Geometry check sheet. Reference: the model listing, model coordinates, mm. Face numbers are marked on the shaded views. A direction names the side the tool comes from. Give positions to 0.01 mm unless a question says otherwise; leave off trailing zeros. Loops run counter-clockwise (first coordinate to the right, second up) from the corner with the lowest first, then second, coordinate; pieces in that order, holes last. Notation, with made-up numbers: (52.5, 56.25) -> (82.5, 56.25) arc R32 ccw to (82.5, 82.25) -> close; hole circle Ø8 at (31.25, 70.5). An arc over 180 degrees is marked (long way). One line per question, with ' | ' between items.
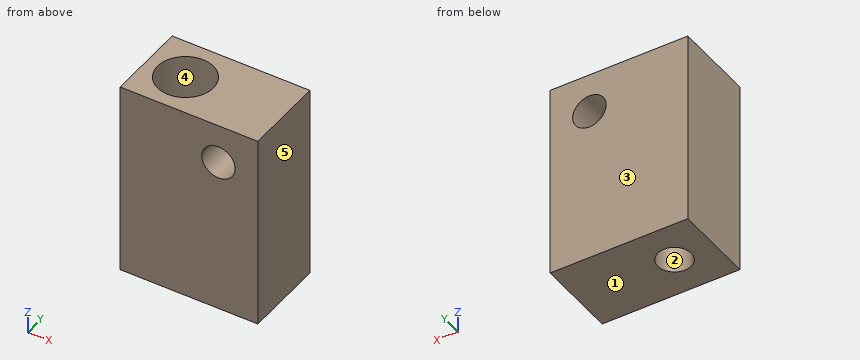
from build123d import *

# Parameters (mm, degrees)
F0_W     = 42
F0_H     = 60
F1_DEPTH = 25
F4_D     = 10.2
F4_DEPTH = 100
F4_TIP   = 3.064389157
F5_D     = 10.2
F5_DEPTH = 100
F5_TIP   = 3.064389157
F6_D     = 17
F6_DEPTH = 35
F6_TIP   = 5.1073152617


with BuildPart() as f1:
    # F0 (on Front) → F1 (new body)
    with BuildSketch(Plane.XZ):
        with Locations((-52.5741710365, 48.0550478399)):
            Rectangle(F0_W, F0_H)
    extrude(amount=F1_DEPTH)

    # F4
    with Locations(Plane.XZ.offset(25)):
        with Locations((-43.5741710365, 66.0550478399)):
            Hole(F4_D / 2, depth=F4_DEPTH)
            with Locations((0, 0, -(F4_DEPTH + F4_TIP / 2))):  # 118° drill point
                Cone(0, F4_D / 2, F4_TIP, mode=Mode.SUBTRACT)

    # F5
    with Locations(Plane.XY.offset(78.0550478399)):
        with Locations((-61.5741710365, -12.5)):
            Hole(F5_D / 2, depth=F5_DEPTH)
            with Locations((0, 0, -(F5_DEPTH + F5_TIP / 2))):  # 118° drill point
                Cone(0, F5_D / 2, F5_TIP, mode=Mode.SUBTRACT)

    # F6
    with Locations(Plane.XY.offset(78.0550478399)):
        with Locations((-61.5741710365, -12.5)):
            Hole(F6_D / 2, depth=F6_DEPTH)
            with Locations((0, 0, -(F6_DEPTH + F6_TIP / 2))):  # 118° drill point
                Cone(0, F6_D / 2, F6_TIP, mode=Mode.SUBTRACT)


solid = f1.part
Item 1: Scan lines: probe 1 along X at (y, z) = (-12.5, 34.25); probe 2 along X at (y, z) = (-12.5, 53.5); probe 3 along X at (y, z) = (-8.25, 69). Record each from-to range of solid material in increasing order.
Result:
probe 1: -73.57 to -66.67, -56.47 to -31.57 | probe 2: -73.57 to -70.07, -53.07 to -31.57 | probe 3: -73.57 to -68.94, -54.21 to -47.74, -39.41 to -31.57
Item 2: Sectioned sample at A-A (y = -12.5). Record the cut outline in (x, z), plus the area to 3 significant figures.
Result:
outline: (-73.57, 18.06) -> (-66.67, 18.06) -> (-66.67, 41.01) -> (-70.07, 43.06) -> (-70.07, 78.06) -> (-73.57, 78.06) -> close; (-56.47, 18.06) -> (-31.57, 18.06) -> (-31.57, 78.06) -> (-53.07, 78.06) -> (-53.07, 43.06) -> (-56.47, 41.01) -> close; hole circle Ø10.2 at (-43.57, 66.06) | area: 1,580 mm2
Item 3: Sectioned sample at C-C (x = -43). Record the cut outline in (y, z), plus the area to 3 significant figures.
Result:
outline: (-25, 18.06) -> (0, 18.06) -> (0, 60.99) -> (-25, 60.99) -> close; (-25, 71.12) -> (0, 71.12) -> (0, 78.06) -> (-25, 78.06) -> close | area: 1,250 mm2
Item 4: Sectioned sample at D-D (z = 31.5). Record the cut outline in (x, y), plus the area to 3 significant figures.
Result:
outline: (-73.57, -25) -> (-31.57, -25) -> (-31.57, 0) -> (-73.57, 0) -> close; hole circle Ø10.2 at (-61.57, -12.5) | area: 968 mm2
Item 5: Release check for a two-part mould opening along Y. For the marked faces 1, 2 and 3 record: pulls with the +Y half, pulls with the -Y half, needs draft (parallel to the pull), parting line crosses it, or undercut.
Result:
face 1: needs draft | face 2: undercut | face 3: pulls with the +Y half
Item 6: Set-up check for the marked faces 4 and 5: record each of +Z, -Z, +X, -X, +Y, -Y from which the full face is reachable in a straight line by a thin tool's end or side.
Result:
face 4: +Z | face 5: +Z, -Z, +X, +Y, -Y
Item 7: Sectioned sample at B-B (z = 52.5). Record the cut outline in (x, y).
Result:
outline: (-73.57, -25) -> (-31.57, -25) -> (-31.57, 0) -> (-73.57, 0) -> close; hole circle Ø17 at (-61.57, -12.5)
